Can you work these out from the drawing? Everything is in mm from the part's minimum corner. A direction names the side the tool comes from. Round coordinates to 2 decimals unless told otherwise and drop trailing zeros. Loops run counter-clockwise (first coordinate to the right, second up) from the corner with the lowest first, then second, coordinate; pieces in that order, holes last. Notation, with made-up numbers: M 9,-32.5 L 46,-32.5 A37 ccw 46,6.5 Z; hole C 15,89.25 d7. An arc over 180 degrees is marked long. Use a Markdown table: item, result.
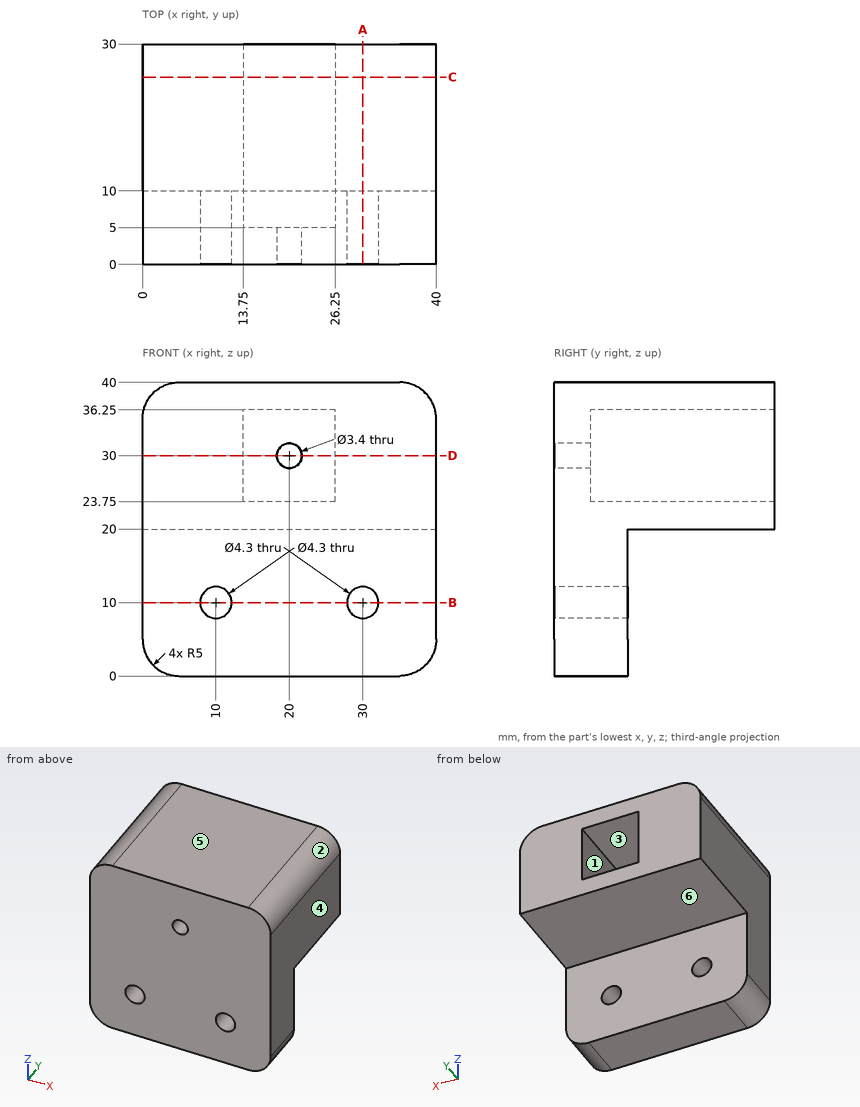
1. I need wall thicknesses on probe 1 along Z at (x, y) = (25, 15.75); probe 2 along Z at (x, y) = (30, 4); probe 3 along X at (y, z) = (1.3, 30). Which ranges of each line are inside material? Lowest first, please. Write a range as from..to.
Answer sheet:
| item | result |
|---|---|
| probe 1 | 20..23.75, 36.25..40 |
| probe 2 | 0..7.85, 12.15..40 |
| probe 3 | 0..18.3, 21.7..40 |
2. Imagine slicing it at C-C, the plane y = 25.5. Write out the boundary of the cut face in (x, z), then the cut area to 3 significant figures.
Answer sheet:
| item | result |
|---|---|
| outline | M 0,20 L 40,20 L 40,35 A5 ccw 35,40 L 5,40 A5 ccw 0,35 Z; hole M 13.75,23.75 L 26.25,23.75 L 26.25,36.25 L 13.75,36.25 Z |
| area | 633 mm2 |
3. Which directions (+Z, -Z, +X, -X, +Y, -Y) give clear straight access to the entire face, cutting with the end or side of a thin tool? Please do the marked faces 5 and 6.
Answer sheet:
| item | result |
|---|---|
| face 5 | +Z, +X, -X, +Y, -Y |
| face 6 | -Z, +X, -X, +Y |
4. For pin 1 Ø5.5 at (x, z) = (10, 10) entering from +Y; pin 2 Ø6 at (x, y) = (18, 20) entering from -Z; pin 3 Ø3.5 at (x, z) = (30, 10) entering from -Y, each with a flat end and sliding along its axis, tell me the tip position at first contact or that it passes through.
Answer sheet:
| item | result |
|---|---|
| pin 1 | y = 10 |
| pin 2 | z = 20 |
| pin 3 | through |
5. We'd pull the mould along Z, two halves only. Please class the marked faces 1, 2, 3 and 4: +Z half, -Z half, draft (parallel to the pull), parting line (faces both ways), or undercut.
Answer sheet:
| item | result |
|---|---|
| face 1 | undercut |
| face 2 | +Z half |
| face 3 | undercut |
| face 4 | draft |
6. Imagine slicing it at A-A, the plane x = 30. Write out the boundary of the cut face in (y, z), then the cut area to 3 significant figures.
Answer sheet:
| item | result |
|---|---|
| outline | M 0,0 L 10,0 L 10,7.85 L 0,7.85 Z; M 0,12.15 L 10,12.15 L 10,20 L 30,20 L 30,40 L 0,40 Z |
| area | 757 mm2 |
7. Imagine slicing it at B-B, the plane z = 10. Write out the boundary of the cut face in (x, y), then the cut area to 3 significant figures.
Answer sheet:
| item | result |
|---|---|
| outline | M 0,0 L 7.85,0 L 7.85,10 L 0,10 Z; M 12.15,0 L 27.85,0 L 27.85,10 L 12.15,10 Z; M 32.15,0 L 40,0 L 40,10 L 32.15,10 Z |
| area | 314 mm2 |
8. Imagine slicing it at D-D, the plane z = 30. Write out the boundary of the cut face in (x, y), then the cut area to 4 significant figures.
Answer sheet:
| item | result |
|---|---|
| outline | M 0,0 L 18.3,0 L 18.3,5 L 13.75,5 L 13.75,30 L 0,30 Z; M 21.7,0 L 40,0 L 40,30 L 26.25,30 L 26.25,5 L 21.7,5 Z |
| area | 870.5 mm2 |
